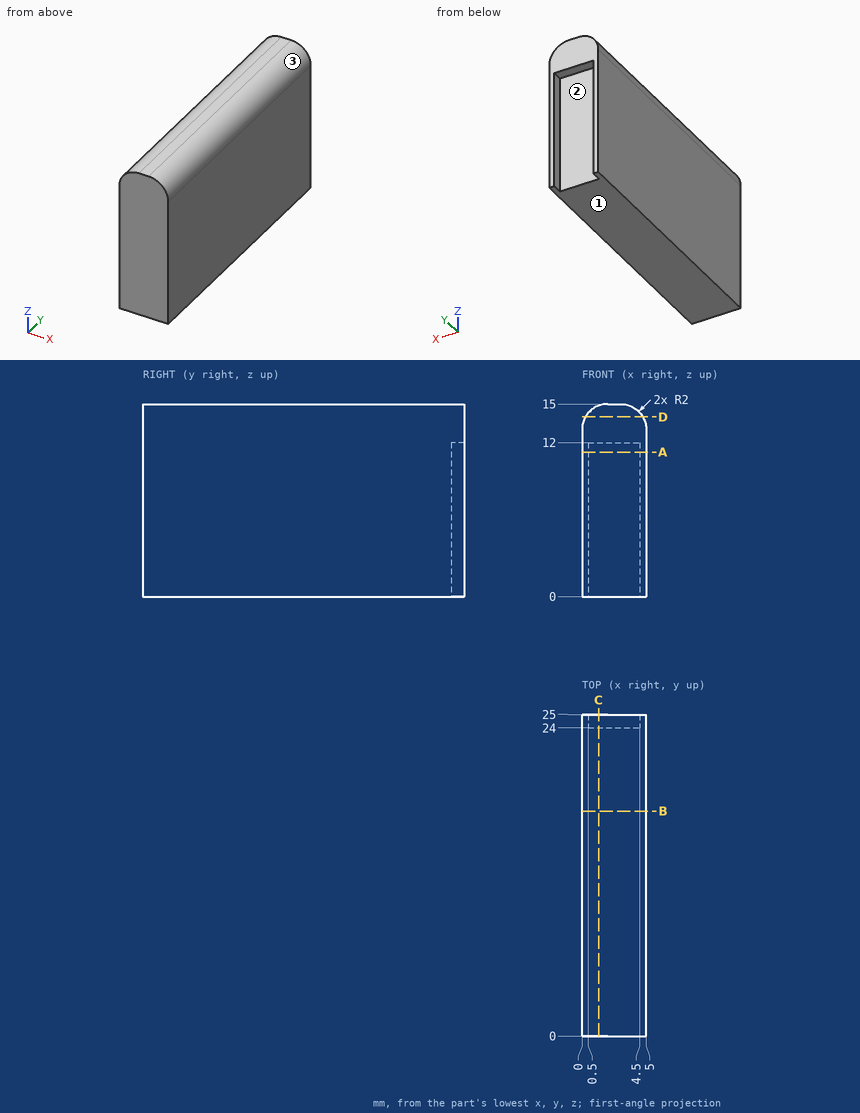
Print and shaded views of the part. All mm, measured from the part's lowest x, y and z. Coordinates: 2 decimals unless noted, no trailing zeros. Order: outer loops, then holes, each group sorted by start corner. A loop starts at its lowest first (then second) coordinate and runs counter-clockwise, first axis right, second up. Notation, with made-up numbers: (18, 19.5) -> (62, 19.5) arc R7 cw to (62, 28.5) -> close; hole circle Ø2 at (-7.75, 60.5). An arc over 180 degrees is marked (long way). Answer as a JSON object with one key per item and string values. Group by question number.
1) Flat gauge pin, fed straight in: pin 1 (0.8 mm diameter, centred on x = 3, y = 24.5, fed in from -Z). Where does the tip first touch, or does it go through?
2) Pull direction X, two halves, no side cores. Call the marked faces 1, 2 and 3: +X half, -X half, draft (parallel to the pull), parting line (faces both ways), or undercut.
3) Drill centre lines: L1, parallel to Y at x = 2.25, z = 9; L2, parallel to Z at x = 3.15, y = 13.5; L3, parallel to Z at x = 0.9, y = 8. Where is each one in solid material? Low to high.
4) Cut at B-B, the plane y = 17.5. Write the cut outline in (x, z).
5) Cut at A-A, the plane z = 11.25. Write the cut outline in (x, y).
6) Cut at D-D, the plane z = 14. Write the cut outline in (x, y).
7) Cut at C-C, the plane x = 1.3. Write the cut outline in (y, z).
Check values:
{
 "1": {"pin 1": "stops at z = 12"},
 "2": {"face 1": "draft", "face 2": "undercut", "face 3": "+X half"},
 "3": {"L1": "y = 0 to 24", "L2": "z = 0 to 14.99", "L3": "z = 0 to 14.67"},
 "4": {"outline": "(0, 0) -> (5, 0) -> (5, 13) arc R2 ccw to (3, 15) -> (2, 15) arc R2 ccw to (0, 13) -> close"},
 "5": {"outline": "(0, 0) -> (5, 0) -> (5, 25) -> (4.5, 25) -> (4.5, 24) -> (0.5, 24) -> (0.5, 25) -> (0, 25) -> close"},
 "6": {"outline": "(0.27, 0) -> (4.73, 0) -> (4.73, 25) -> (0.27, 25) -> close"},
 "7": {"outline": "(0, 0) -> (24, 0) -> (24, 12) -> (25, 12) -> (25, 14.87) -> (0, 14.87) -> close"}
}
